Build history of the part. All positions in model axes, mm. Face numbers are marked on the shaded views. A direction names the side the tool comes from. Round coordinates to 2 decimals unless told otherwise and drop trailing zeros. Loops run counter-clockwise (first coordinate to the right, second up) from the corner with the lowest first, then second, coordinate; pieces in that order, holes last. Notation, with made-up numbers: (15, 49) -> (57, 49) arc R10 cw to (57, 58) -> close; hole circle Ø4 at (29.25, 84). An arc over 180 degrees is marked (long way). Put each result on its own line as item: value. Start each with the question number.
Item 1: Flat gauge pins, fed straight in: pin 1 Ø2 at (y, z) = (-0.5, 6.5) entering from -X; pin 2 Ø2 at (y, z) = (-3, 10) entering from -X; pin 3 Ø2 at (x, z) = (1.5, -2.5) entering from +Y. Where does each tip first touch, or does it go through?
Item 2: Tool access for the marked faces 4 and 5: list every direction of +Z, -Z, +X, -X, +Y, -Y with a clear straight run to the whole face (end or side of a thin tool).
Item 3: Pull direction Y, two halves, no side cores. Call the marked faces 1, 2 and 3: +Y half, -Y half, draft (parallel to the pull), parting line (faces both ways), or undercut.
Item 4: Drill centre lines: probe 1 along Z at (x, y) = (-2.25, 2); probe 2 along Z at (x, y) = (1.75, 0.5); probe 3 along Z at (x, y) = (1.5, 0.25). Where is each one in solid material? Low to high. Write a range as [from, to].
Item 5: Cut at A-A, the plane z = -6.5. List the corners of the cut face in (x, y).
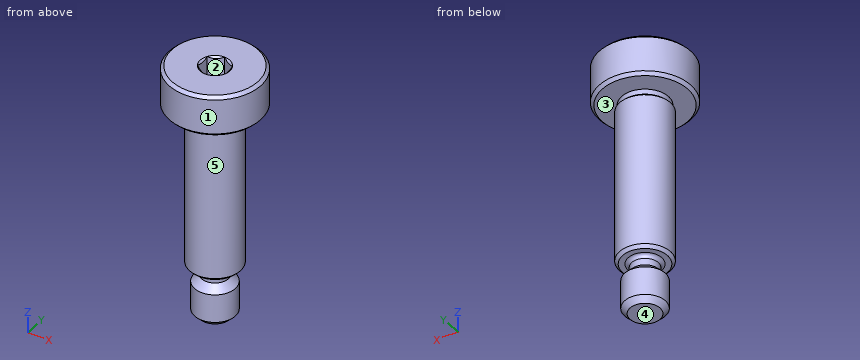
```python
from build123d import *

# Parameters (mm, degrees)
CUT_EXTRUDE1_START = 12.5
CUT_EXTRUDE1_DEPTH = 2
CHAMFER1_SIZE      = 0.2925


with BuildPart() as part:
    # Sketch3 → Revolve1 (revolve)
    with BuildSketch(Plane(origin=(0, 0, 0), x_dir=(0, 0, -1), z_dir=(1, 0, 0)), mode=Mode.PRIVATE) as revolve1_sk:
        with BuildLine():
            Line((-12.5, 0), (-12.5, 4.2075))
            Line((-12.5, 4.2075), (-12.2075, 4.5))
            Line((-12.2075, 4.5), (-8.7925, 4.5))
            Line((-8.7925, 4.5), (-8.5, 4.2075))
            Line((-8.5, 4.2075), (-8.5, 2.297))
            Line((-8.5, 2.297), (-7.992, 2.297))
            Line((-7.992, 2.297), (-7.789, 2.5))
            Line((-7.789, 2.5), (7.5, 2.5))
            Line((7.5, 2.5), (7.5, 1.65))
            ThreePointArc((7.5, 1.65), (7.602512627, 1.402512627), (7.85, 1.3))
            Line((7.85, 1.3), (8.5, 1.3))
            Line((8.5, 1.3), (9.2, 2))
            Line((9.2, 2), (11.975, 2))
            Line((11.975, 2), (12.5, 1.475))
            Line((12.5, 1.475), (12.5, 0))
            Line((12.5, 0), (-12.5, 0))
        make_face()
    revolve(revolve1_sk.sketch.rotate(Axis((0, 0, 12.5), (0, 0, -1)), 90), axis=Axis((0, 0, 12.5), (0, 0, -1)))

    # Sketch4 → Cut-Extrude1 (cut)
    with BuildSketch(Plane.XY.offset(CUT_EXTRUDE1_START)):
        Polygon((0, 1.443375673), (-1.25, 0.721687836), (-1.25, -0.721687836), (0, -1.443375673), (1.25, -0.721687836), (1.25, 0.721687836), align=None)
    extrude(amount=-CUT_EXTRUDE1_DEPTH, mode=Mode.SUBTRACT)

    # Cut-Extrude2 cone 1 section (through the dimple's axis) → Cut-Extrude2 (revolve, cut)
    with BuildSketch(Plane(origin=(0, 0, 12.5), x_dir=(0, -1, 0), z_dir=(1, 0, 0))):
        Polygon((0, 0), (1.443375673, 0), (0, 1.443375673), align=None)
    revolve(axis=Axis((0, 0, 12.5), (0, 0, -1)), mode=Mode.SUBTRACT)

    # Chamfer1
    chamfer1_edges = [part.edges().sort_by_distance(p)[0] for p in [
        (-2.5, 0, -7.5),
    ]]
    chamfer(chamfer1_edges, length=CHAMFER1_SIZE)


solid = part.part
```
Reply:
1. pin 1: stops at x = -2.5
1. pin 2: stops at x = -4.03
1. pin 3: stops at y = 2.45
2. face 4: -Z, +X, -X, +Y, -Y
2. face 5: -Z
3. face 1: parting line
3. face 2: undercut
3. face 3: draft
4. probe 1: z = [8.5, 12.5]
4. probe 2: z = [-12.15, -9.02], [-7.5, 12.5]
4. probe 3: z = [-12.45, -8.72], [-7.52, 12.5]
5. outline: circle Ø5 at (0, 0)
